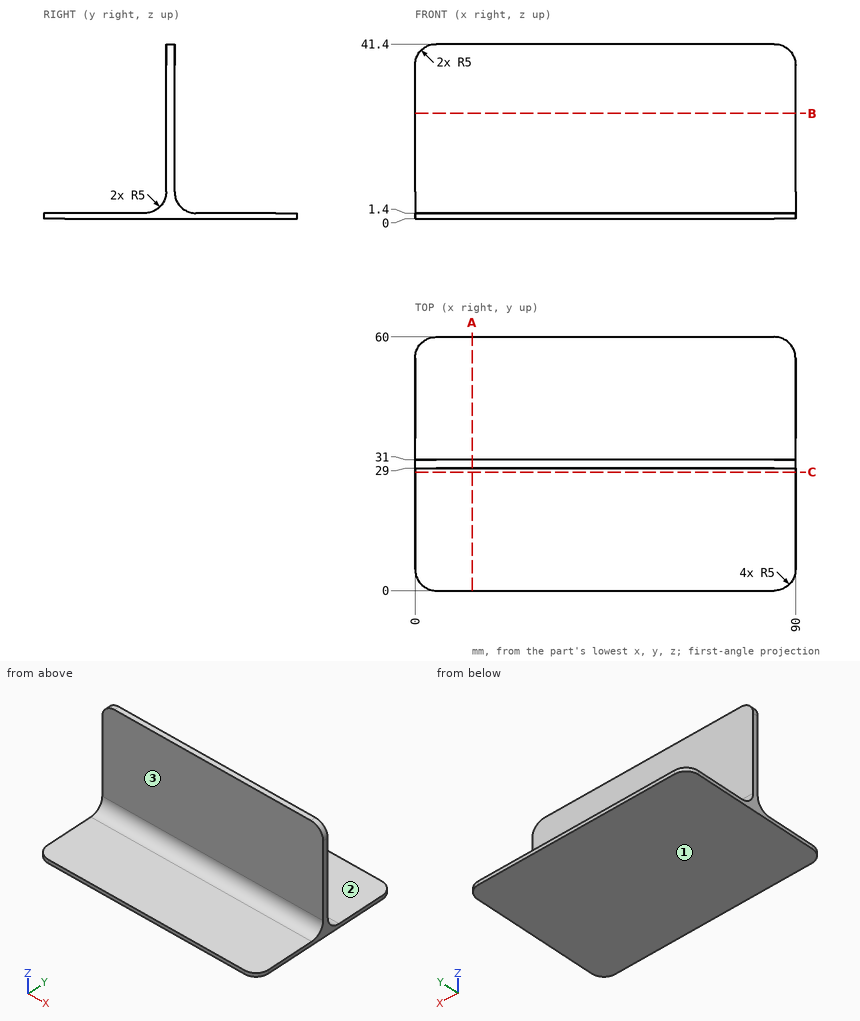
Drawing for the job (mm, zero at the part's lowest x, y, z). A direction names the side the tool comes from. Round coordinates to 2 decimals unless told otherwise and drop trailing zeros. Loops run counter-clockwise (first coordinate to the right, second up) from the corner with the lowest first, then second, coordinate; pieces in that order, holes last. Notation, with made-up numbers: (44, 24.25) -> (59, 24.25) arc R35 cw to (59, 58.25) -> close; hole circle Ø9 at (39.5, -28). An arc over 180 degrees is marked (long way). Answer in a Markdown table with one row per item.
Item 1: Which spindle directions (+Z, -Z, +X, -X, +Y, -Y) get a long thin tool onto all of the face, cutting with end or side? Do the marked faces 1, 2 and 3. Say none if no direction does.
Answers below:
| item | result |
|---|---|
| face 1 | -Z, +X, -X, +Y, -Y |
| face 2 | +Z, +X, -X, +Y |
| face 3 | +Z, +X, -X, -Y |
Item 2: Drill centre lines: L1, parallel to Y at x = 38.5, z = 16; L2, parallel to Z at x = 73, y = 42.5; L3, parallel to Y at x = 21, z = 2.5. Where is each one in solid material? Low to high. Write a range as [from, to].
Answers below:
| item | result |
|---|---|
| L1 | y = [29, 31] |
| L2 | z = [0, 1.4] |
| L3 | y = [27.13, 32.87] |
Item 3: Saw through at C-C (y = 28). Write the cut outline in (x, z), and give its area (3 significant figures).
Answers below:
| item | result |
|---|---|
| outline | (0, 0) -> (90, 0) -> (90, 3.4) -> (0, 3.4) -> close |
| area | 306 mm² |
Item 4: Saw through at B-B (z = 25). Write the cut outline in (x, y).
Answers below:
| item | result |
|---|---|
| outline | (0, 29) -> (90, 29) -> (90, 31) -> (0, 31) -> close |
Item 5: Pin check, flat tips, straight feed: pin 1 (19 mm diameter, centred on x = 43.5, y = 9.5, fed in from +Z); pin 2 (8 mm diameter, centred on x = 52, y = 36.5, fed in from +Z); pin 3 (1 mm diameter, centred on x = 48.5, z = 35.5, fed in from -Y). Stop position of each tip, or through.
Answers below:
| item | result |
|---|---|
| pin 1 | stops at z = 1.4 |
| pin 2 | stops at z = 2.83 |
| pin 3 | stops at y = 29 |
Item 6: Saw through at A-A (x = 13.5). Write the cut outline in (y, z).
Answers below:
| item | result |
|---|---|
| outline | (0, 0) -> (60, 0) -> (60, 1.4) -> (36, 1.4) arc R5 cw to (31, 6.4) -> (31, 41.4) -> (29, 41.4) -> (29, 6.4) arc R5 cw to (24, 1.4) -> (0, 1.4) -> close |
